Part model, mm, in its own coordinate system. A direction names the side the tool comes from. Give positions to 0.01 mm unless a question says otherwise; leave off trailing zeros. Order: outer loops, then holes, each group sorted by start corner. A loop starts at its lowest first (then second) coordinate and runs counter-clockwise, first axis right, second up. Notation, with made-up numbers: (46.25, -32.75) - (66.25, -32.75) arc R12 cw to (66.25, -21.75) - close; hole circle Ø4 at (44, 76). An arc over 180 degrees is marked (long way). One line per item, written item: value.
Autodesk Fusion 360 part; units mm, degrees
sketch "air pipe clamp base" plane through (0, 0, 0) normal (0, 0, 1) x (1, 0, 0)
  line L0 (-6.5, -9.2601) -> (-6.5, -16.5993)
  line L1 (-6.5, -16.5993) -> (-2.5, -16.5993)
  line L2 (2.5, -16.5993) -> (6.5, -16.5993)
  line L3 (6.5, -16.5993) -> (6.5, -9.2601)
  line L4 (-2.5, -16.5993) -> (-2.5, -7.5993)
  line L5 (2.5, -16.5993) -> (2.5, -7.5993)
  arc A0 (7.5, -6.6144) -> (-7.5, -6.6144) centre (0, 0) ccw
  arc A1 (3.9, -4.5596) -> (-3.9, -4.5596) centre (0, 0) ccw
  line L6 (0, 0) -> (0, -19.8599) construction
  arc A2 (-2.5, -7.5993) -> (-3.9, -4.5596) centre (-6.5, -7.5993) ccw
  arc A3 (3.9, -4.5596) -> (2.5, -7.5993) centre (6.5, -7.5993) ccw
  arc A4 (-6.5, -9.2601) -> (-7.5, -6.6144) centre (-10.5, -9.2601) ccw
  arc A5 (7.5, -6.6144) -> (6.5, -9.2601) centre (10.5, -9.2601) ccw
  point P0 (-6.5, -7.5993)
  dimension "d1" = 12
  dimension "d3" = 4
  dimension "d4" = 5
  dimension "d5" = 4
  dimension "d6" = 4
  dimension "d7" = 9
  dimension "d8" = 4
extrude "Extrude1" add sketch "air pipe clamp base" along normal blind 10
sketch "screw holes" plane through (-6.5, 0, 0) normal (-1, 0, 0) x (0, 0, 1)
  line L0 (0, -9.2601) -> (0, -16.5993)
  line L1 (0, -16.5993) -> (10, -16.5993)
  line L2 (10, -16.5993) -> (10, -9.2601)
  line L3 (10, -9.2601) -> (0, -9.2601)
  line L4 (0, -9.2601) -> (10, -16.5993) construction
  line L5 (10, -9.2601) -> (0, -16.5993) construction
  point P0 (5, -12.9297)
hole "Hole1" at (-6.5, -12.9297, 5) direction (1, 0, 0) diameter 4.7 depth 5 tip angle 180
hole "Hole2" at (-6.5, -12.9297, 5) direction (1, 0, 0) diameter 3.3 depth 25 tip angle 180
fillet "Fillet1" radius 0.6 4 edges at (-6.5, -16.5993, 5) (-2.5, -16.5993, 5) (2.5, -16.5993, 5) (6.5, -16.5993, 5)
chamfer "Chamfer1" distance 0.4 angle 45 2 faces at (-3.8333, -10.9529, 10) (-3.8333, -10.9529, 0)
1) Pin check, flat tips, straight feed: pin 1 (10 mm diameter, centred on x = 2, y = -2, fed in from +Z); pin 2 (2.5 mm diameter, centred on y = -10, z = 5.5, fed in from -X); pin 3 (4 mm diameter, centred on y = 4.5, z = 3, fed in from +X); pin 4 (2 mm diameter, centred on y = -12, z = 5.5, fed in from +X). Stop position of each tip, or through.
Outcome:
pin 1: stops at z = 10
pin 2: stops at x = -6.53
pin 3: stops at x = 9.68
pin 4: stops at x = 6.5
2) Which spindle directions (+Z, -Z, +X, -X, +Y, -Y) get a long thin tool onto all of the face, cutting with end or side? Do faces 4 (the flat face through (6.5, -11, 5)), 5 (the cylindrical face through (-2.88, -5.9, 4.94)), 6 (the flat face through (2.5, -11, 5)), 7 (the flat face through (-6.5, -10, 5)). Say none if no direction does.
Outcome:
face 4: +Z, -Z, +X, -Y
face 5: +Z, -Z
face 6: +Z, -Z, -Y
face 7: +Z, -Z, -X, -Y
3) Cut at B-B, the plane z = 5. Give the cut face in (x, y), then the cut area to 3 significant figures.
Outcome:
outline: (-7.5, -6.61) arc R4 cw to (-6.5, -9.26) - (-6.5, -10.58) - (-2.5, -10.58) - (-2.5, -7.6) arc R4 ccw to (-3.9, -4.56) arc R6 cw (long way) to (3.9, -4.56) arc R4 ccw to (2.5, -7.6) - (2.5, -11.28) - (6.5, -11.28) - (6.5, -9.26) arc R4 cw to (7.5, -6.61) arc R10 ccw (long way) to start; (-6.5, -16) arc R0.6 ccw to (-5.9, -16.6) - (-3.1, -16.6) arc R0.6 ccw to (-2.5, -16) - (-2.5, -15.28) - (-6.5, -15.28) - close; (2.5, -16) arc R0.6 ccw to (3.1, -16.6) - (5.9, -16.6) arc R0.6 ccw to (6.5, -16) - (6.5, -14.58) - (2.5, -14.58) - close
area: 210 mm^2
4) Mould opens along Z. For faces 1 (the flat face through (-7, 0, 10)), 2 (the cylindrical face through (-4.47, -13.64, 7.24)), 3 (the cylindrical face through (2.857, -5.948, 4.936)) say: released by +Z, released by -Z, zero draft, split by the parting line, or undercut.
Outcome:
face 1: released by +Z
face 2: undercut
face 3: zero draft
5) Cut at C-C, the plane z = 3. Give the cut face in (x, y).
Outcome:
outline: (-7.5, -6.61) arc R4 cw to (-6.5, -9.26) - (-6.5, -11.7) - (-2.5, -11.7) - (-2.5, -7.6) arc R4 ccw to (-3.9, -4.56) arc R6 cw (long way) to (3.9, -4.56) arc R4 ccw to (2.5, -7.6) - (2.5, -16) arc R0.6 ccw to (3.1, -16.6) - (5.9, -16.6) arc R0.6 ccw to (6.5, -16) - (6.5, -9.26) arc R4 cw to (7.5, -6.61) arc R10 ccw (long way) to start; (-6.5, -16) arc R0.6 ccw to (-5.9, -16.6) - (-3.1, -16.6) arc R0.6 ccw to (-2.5, -16) - (-2.5, -14.16) - (-6.5, -14.16) - close
6) Drill centre lines: line 1 along X through (y, z) = (-12.5, 8); line 2 along X through (y, z) = (0, 5.5); line 3 along Y through (x, z) = (-4.5, 3.5). Where is each one in solid material? Low to high. Write a range as from..to.
Outcome:
line 1: x = -6.5..-2.5, 2.5..6.5
line 2: x = -10..-6, 6..10
line 3: y = -16.6..-14.74, -11.12..-3.97, 3.97..8.93
7) Cut at A-A, the plane y = 0. Give the cut face in (x, z), then the cut area to 3 significant figures.
Outcome:
outline: (-10, 0.4) - (-9.6, 0) - (-6.4, 0) - (-6, 0.4) - (-6, 9.6) - (-6.4, 10) - (-9.6, 10) - (-10, 9.6) - close; (6, 0.4) - (6.4, 0) - (9.6, 0) - (10, 0.4) - (10, 9.6) - (9.6, 10) - (6.4, 10) - (6, 9.6) - close
area: 79.4 mm^2
8) Cut at D-D, the plane x = 0. Give the cut face in (y, z).
Outcome:
outline: (6, 0.4) - (6.4, 0) - (9.6, 0) - (10, 0.4) - (10, 9.6) - (9.6, 10) - (6.4, 10) - (6, 9.6) - close
